```python
from build123d import *

# Parameters (mm, degrees)
BOSS_EXTRUDE1_DEPTH = 711.2
REVOLVE13_ANGLE     = 90
REVOLVE12_ANGLE     = 90
BOSS_EXTRUDE3_DEPTH = 711.2
REVOLVE2_ANGLE      = 90
SKETCH9_R           = 31.75
BOSS_EXTRUDE4_DEPTH = 711.2
REVOLVE10_ANGLE     = 90
BOSS_EXTRUDE5_DEPTH = 711.2


with BuildPart() as part:
    # Sketch1 → Boss-Extrude1 (new body)
    with BuildSketch(Plane(origin=(0, 0, 0), x_dir=(0, 0, -1), z_dir=(1, 0, 0))):
        with BuildLine():
            Line((-31.75, 0), (-31.75, -63.5))
            ThreePointArc((-31.75, -63.5), (-22.450640303, -85.950640303), (0, -95.25))
            Line((0, -95.25), (31.75, -95.25))
            Line((31.75, -95.25), (31.75, 0))
            Line((31.75, 0), (31.75, 31.75))
            Line((31.75, 31.75), (0, 31.75))
            ThreePointArc((0, 31.75), (-22.450640303, 22.450640303), (-31.75, 0))
        make_face()
    extrude(amount=BOSS_EXTRUDE1_DEPTH)



with BuildPart() as body_2:
    # Sketch8 → Revolve13 (revolve)
    with BuildSketch(Plane(origin=(711.2, 0, 0), x_dir=(0, 0, -1), z_dir=(1, 0, 0))):
        with BuildLine():
            Line((-31.75, 0), (-31.75, -63.5))
            ThreePointArc((-31.75, -63.5), (-22.450640303, -85.950640303), (0, -95.25))
            Line((0, -95.25), (31.75, -95.25))
            Line((31.75, -95.25), (31.75, 31.75))
            Line((31.75, 31.75), (0, 31.75))
            ThreePointArc((0, 31.75), (-22.450640303, 22.450640303), (-31.75, 0))
        make_face()
    revolve(axis=Axis((711.2, -95.25, -31.75), (0, 1, 0)), revolution_arc=REVOLVE13_ANGLE)


with BuildPart() as body_3:
    # Sketch15 → Revolve12 (revolve)
    with BuildSketch(Plane(origin=(0, 0, -31.75), x_dir=(0, 0, 1), z_dir=(-1, 0, 0))):
        with BuildLine():
            Line((63.5, -63.5), (63.5, 0))
            ThreePointArc((63.5, 0), (54.200640303, 22.450640303), (31.75, 31.75))
            Line((31.75, 31.75), (0, 31.75))
            Line((0, 31.75), (0, -95.25))
            Line((0, -95.25), (31.75, -95.25))
            ThreePointArc((31.75, -95.25), (54.200640303, -85.950640303), (63.5, -63.5))
        make_face()
    revolve(axis=Axis((0, 31.75, -31.75), (0, -1, 0)), revolution_arc=REVOLVE12_ANGLE)


with BuildPart() as part_1:
    add(part.part)

    add(body_2.part)  # Boss-Extrude3 merges body 2
    # Sketch7 → Boss-Extrude3 (add)
    with BuildSketch(Plane(origin=(0, 0, -31.75), x_dir=(-1, 0, 0), z_dir=(0, 0, -1))):
        with BuildLine():
            Line((-774.7, 0), (-774.7, -63.5))
            ThreePointArc((-774.7, -63.5), (-765.400640303, -85.950640303), (-742.95, -95.25))
            Line((-742.95, -95.25), (-711.2, -95.25))
            Line((-711.2, -95.25), (-711.2, 31.75))
            Line((-711.2, 31.75), (-742.95, 31.75))
            ThreePointArc((-742.95, 31.75), (-765.400640303, 22.450640303), (-774.7, 0))
        make_face()
    extrude(amount=BOSS_EXTRUDE3_DEPTH)

    # Sketch12 → Revolve2 (revolve)
    with BuildSketch(Plane(origin=(1454.15, 0, -742.95), x_dir=(-1, 0, 0), z_dir=(0, 0, -1))):
        with BuildLine():
            Line((679.45, 0), (679.45, -63.5))
            ThreePointArc((679.45, -63.5), (688.749359697, -85.950640303), (711.2, -95.25))
            Line((711.2, -95.25), (742.95, -95.25))
            Line((742.95, -95.25), (742.95, 31.75))
            Line((742.95, 31.75), (711.2, 31.75))
            ThreePointArc((711.2, 31.75), (688.749359697, 22.450640303), (679.45, 0))
        make_face()
    revolve(axis=Axis((711.2, -95.25, -742.95), (0, 1, 0)), revolution_arc=REVOLVE2_ANGLE)


    add(body_3.part)  # Boss-Extrude4 merges body 3
    # Sketch9 → Boss-Extrude4 (add)
    with BuildSketch(Plane(origin=(0, 0, -31.75), x_dir=(-1, 0, 0), z_dir=(0, 0, -1))):
        with BuildLine():
            ThreePointArc((0, 4.4e-08), (9.299359713, 22.450640318), (31.75, 31.75))
            Line((31.75, 31.75), (0, 31.75))
            Line((0, 31.75), (0, 4.4e-08))
        make_face()
        with Locations((31.75, 0)):
            Circle(SKETCH9_R)
        with BuildLine():
            ThreePointArc((31.75, -31.75), (9.299359682, -22.450640287), (0, 4.4e-08))
            Line((0, 4.4e-08), (0, -63.500000004))
            ThreePointArc((0, -63.500000004), (9.299359696, -41.049359699), (31.75, -31.75))
        make_face()
        with BuildLine():
            Line((63.5, -63.5), (63.5, 0))
            ThreePointArc((63.5, 0), (54.200640303, -22.450640303), (31.75, -31.75))
            ThreePointArc((31.75, -31.75), (54.200640303, -41.049359697), (63.5, -63.5))
        make_face()
        with Locations((31.75, -63.5)):
            Circle(SKETCH9_R)
        with BuildLine():
            ThreePointArc((31.75, -95.25), (9.299359699, -85.950640304), (0, -63.500000004))
            Line((0, -63.500000004), (0, -95.25))
            Line((0, -95.25), (31.75, -95.25))
        make_face()
    extrude(amount=BOSS_EXTRUDE4_DEPTH)


with BuildPart() as body_2_2:
    # Sketch14 → Revolve10 (revolve)
    with BuildSketch(Plane(origin=(0, 0, -742.95), x_dir=(-1, 0, 0), z_dir=(0, 0, -1))):
        with BuildLine():
            Line((31.75, 31.75), (0, 31.75))
            Line((0, 31.75), (0, -95.25))
            Line((0, -95.25), (31.75, -95.25))
            ThreePointArc((31.75, -95.25), (54.200640303, -85.950640303), (63.5, -63.5))
            Line((63.5, -63.5), (63.5, 0))
            ThreePointArc((63.5, 0), (54.200640303, 22.450640303), (31.75, 31.75))
        make_face()
    revolve(axis=Axis((0, 31.75, -742.95), (0, -1, 0)), revolution_arc=REVOLVE10_ANGLE)


with BuildPart() as body_3_2:
    # Sketch10 → Boss-Extrude5 (new body)
    with BuildSketch(Plane(origin=(0, 0, 0), x_dir=(0, 0, -1), z_dir=(1, 0, 0))):
        with BuildLine():
            Line((774.7, 31.75), (742.95, 31.75))
            Line((742.95, 31.75), (742.95, -95.25))
            Line((742.95, -95.25), (774.7, -95.25))
            ThreePointArc((774.7, -95.25), (797.150640303, -85.950640303), (806.45, -63.5))
            Line((806.45, -63.5), (806.45, 0))
            ThreePointArc((806.45, 0), (797.150640303, 22.450640303), (774.7, 31.75))
        make_face()
    extrude(amount=BOSS_EXTRUDE5_DEPTH)


with BuildPart() as part_2:
    add(part_1.part)

    # Combine1: union body 3 2, body 2 2
    add(body_3_2.part)
    add(body_2_2.part)


solid = part_2.part
```
Verification items for the finished model (mm, model axes). A direction names the side the tool comes from. Coordinates: 2 decimals unless noted, no trailing zeros. Write each loop counter-clockwise with the first axis right and the second up, starting at its lowest first coordinate (ties: lowest second). Pieces come first, ordered by that corner, then holes. Notation, with made-up numbers: (6, 88) - (64, 88) arc R29 cw to (64, 123) - close; hole circle Ø7 at (85.25, 3.25). An arc over 180 degrees is marked (long way). Write item = value, one per line.
Q1. Cross-section at B-B (x = 109.5). Enter the section's corners in (y, z).
Answer:
outline = (-95.25, -774.7) arc R31.75 ccw to (-63.5, -806.45) - (0, -806.45) arc R31.75 ccw to (31.75, -774.7) - (31.75, -742.95) - (-95.25, -742.95) - close; (-95.25, -31.75) - (31.75, -31.75) - (31.75, 0) arc R31.75 ccw to (0, 31.75) - (-63.5, 31.75) arc R31.75 ccw to (-95.25, 0) - close
Q2. Cross-section at D-D (y = -81). Enter the section's corners in (x, z).
Answer:
outline = (-58.24, -742.95) arc R58.24 ccw to (0, -801.19) - (711.2, -801.19) arc R58.24 ccw to (769.44, -742.95) - (769.44, -31.75) arc R58.24 ccw to (711.2, 26.49) - (0, 26.49) arc R58.24 ccw to (-58.24, -31.75) - close; hole (0, -742.95) - (711.2, -742.95) - (711.2, -31.75) - (0, -31.75) - close
Q3. Material ranges on L1, parallel to X at y = -3, z = -181.5; L2, parallel to Z at x = 586.5, y = -59; L3, parallel to Z at x = 285.5, y = 1.5, recorded low to high. Write a range as from..to.
Answer:
L1 = -63.5..0, 711.2..774.7
L2 = -806.45..-742.95, -31.75..31.75
L3 = -806.41..-742.95, -31.75..31.71
Q4. Cross-section at A-A (z = -99.5). Enter the section's corners in (x, y), plus the area to 3 significant figures.
Answer:
outline = (-63.5, -63.5) arc R31.75 ccw to (-31.75, -95.25) - (0, -95.25) - (0, 31.75) - (-31.75, 31.75) arc R31.75 ccw to (-63.5, 0) - close; (711.2, -95.25) - (742.95, -95.25) arc R31.75 ccw to (774.7, -63.5) - (774.7, 0) arc R31.75 ccw to (742.95, 31.75) - (711.2, 31.75) - close
area = 15,300 mm²
Q5. Go/stop test with a flat-tipped pin: pin 1 Ø8 at (y, z) = (-76.5, -440) entering from -X. Record where the tip stops, or that it passes through.
Answer:
pin_1 = -62.2
Q6. Access from +Z, -Z, +X, -X, +Y, -Y to the whole of each face (thin tool, end or side, straight path). Record for faces 5 (the face through (-45.392, -31.306, -787.355)), 6 (the face through (361, -31, -31.75)).
Answer:
face_5 = -Z, -X, +Y, -Y
face_6 = +Y, -Y
Q7. Cross-section at C-C (y = -17.5). Enter the section's corners in (x, z), plus the area to 3 significant figures.
Answer:
outline = (-63.5, -742.95) arc R63.5 ccw to (0, -806.45) - (711.2, -806.45) arc R63.5 ccw to (774.7, -742.95) - (774.7, -31.75) arc R63.5 ccw to (711.2, 31.75) - (0, 31.75) arc R63.5 ccw to (-63.5, -31.75) - close; hole (0, -742.95) - (711.2, -742.95) - (711.2, -31.75) - (0, -31.75) - close
area = 193,000 mm²
Q8. Mould release check, pull along Z, two halves, no side actions. Record for faces 1 (the face through (0, -31, -382)), 2 (the face through (350.6, -86.2, -796.9)), 3 (the face through (765.65, -85.7, -382.37)), 4 (the face through (350.6, -85.7, 22.7)): released by +Z, released by -Z, zero draft, split by the parting line, or undercut.
Answer:
face_1 = undercut
face_2 = released by -Z
face_3 = zero draft
face_4 = released by +Z
